Read the model definition and answer for the solid it produces. Units are mm, in the model's axes. A direction names the side the tool comes from. Give positions to 0.01 mm unless a question says otherwise; leave off trailing zeros. Write each loop counter-clockwise with the first axis right and the second up, starting at its lowest first coordinate (ties: lowest second). Pieces come first, ordered by that corner, then holes. Notation, with made-up numbers: M 26,-33 L 62,-33 A20 ccw 62,-17 Z; hole C 43.25,-17 d9. An arc over 180 degrees is marked long. Put each result on its own line as item: value.
from build123d import *

# Parameters (mm, degrees)
BOSS_EXTRUDE1_DEPTH = 10
SKETCH2_R           = 3
CUT_EXTRUDE1_DEPTH  = 34
SKETCH3_W           = 8.31174776
SKETCH3_H           = 3.43251071
BOSS_EXTRUDE2_DEPTH = 40
SKETCH4_R           = 2.5
CUT_EXTRUDE2_DEPTH  = 9.963348995


with BuildPart() as part:
    # Sketch1 → Boss-Extrude1 (new body)
    with BuildSketch(Plane.XY):
        with BuildLine():
            Line((0, 0), (38.333333333, 0))
            ThreePointArc((38.333333333, 0), (39.914472163, -0.25658351), (41.333333333, -1))
            Line((41.333333333, -1), (78.666666667, -29))
            ThreePointArc((78.666666667, -29), (80.085527837, -29.74341649), (81.666666667, -30))
            Line((81.666666667, -30), (100, -30))
            Line((100, -30), (100, -33))
            Line((100, -33), (81.666666667, -33))
            ThreePointArc((81.666666667, -33), (79.136844539, -32.589466384), (76.866666667, -31.4))
            Line((76.866666667, -31.4), (39.533333333, -3.4))
            ThreePointArc((39.533333333, -3.4), (38.965788865, -3.102633404), (38.333333333, -3))
            Line((38.333333333, -3), (0, -3))
            Line((0, -3), (0, 0))
        make_face()
    extrude(amount=BOSS_EXTRUDE1_DEPTH)

    # Sketch2 → Cut-Extrude1 (cut, through all)
    with BuildSketch(Plane(origin=(0, 0, 0), x_dir=(1, 0, 0), z_dir=(0, 1, 0))):
        with Locations((6.267592097, -5)):
            Circle(SKETCH2_R)
        with Locations((31.216017877, -5)):
            Circle(SKETCH2_R)
        with Locations((89.111430709, -5)):
            Circle(SKETCH2_R)
    extrude(amount=-CUT_EXTRUDE1_DEPTH, mode=Mode.SUBTRACT)

    # Sketch3 → Boss-Extrude2 (add)
    with BuildSketch(Plane.XZ.offset(33)):
        with Locations((95.527410175, 7.24709364)):
            Rectangle(SKETCH3_W, SKETCH3_H)
    extrude(amount=BOSS_EXTRUDE2_DEPTH)

    # Sketch4 → Cut-Extrude2 (cut, through all)
    with BuildSketch(Plane.XY.offset(8.963348995)):
        with Locations((95.527410175, -67.614542538)):
            Circle(SKETCH4_R)
    extrude(amount=-CUT_EXTRUDE2_DEPTH, mode=Mode.SUBTRACT)


solid = part.part
(1) Section A-A on z = 3.25 is taken. Determine the outline of the cut face in (x, y).
Result:
outline: M 0,-3 L 3.83,-3 L 3.83,0 L 0,0 Z; M 8.7,-3 L 28.78,-3 L 28.78,0 L 8.7,0 Z; M 33.65,-3 L 38.33,-3 A2 cw 39.53,-3.4 L 76.87,-31.4 A8 ccw 81.67,-33 L 86.67,-33 L 86.67,-30 L 81.67,-30 A5 cw 78.67,-29 L 41.33,-1 A5 ccw 38.33,0 L 33.65,0 Z; M 91.55,-33 L 100,-33 L 100,-30 L 91.55,-30 Z
(2) Section B-B on x = 89 is taken. Determine the outline of the cut face in (y, z).
Result:
outline: M -33,0 L -30,0 L -30,2 L -33,2 Z; M -33,8 L -30,8 L -30,10 L -33,10 Z
(3) Given pin 1 Ø0.6 at (x, z) = (92, 6) entering from +Y; pin 2 Ø9 at (x, y) = (96.5, -49) entering from -Z; pin 3 Ø3 at (y, z) = (-28, 6.5) entering from +X, each flat-ended and moving along its own axis, determine where each tip first touches the part or whether it passes through.
Result:
pin 1: stops at y = -30
pin 2: stops at z = 5.53
pin 3: stops at x = 79.49
(4) Straight lines are drawn through the part: line 1 along X through (y, z) = (-1.05, 5); line 2 along Y through (x, z) = (24, 5.75); line 3 along X through (y, z) = (-1.95, 5). For each, find the intervals that lie inside material, in ascending order. Write a range as from..to.
Result:
line 1: x = 0..3.27, 9.27..28.22, 34.22..41.4
line 2: y = -3..0
line 3: x = 0..3.27, 9.27..28.22, 34.22..42.6
(5) Which of the six approach directions +Z, -Z, +X, -X, +Y, -Y give full straight-line access (tool end or side, diameter ignored) to faces 1 (the face through (95, -53, 8.963)), 2 (the face through (99.683, -53, 7)), 3 (the face through (95, -53, 5.531)), 4 (the face through (93, -30, 5))?
Result:
face 1: +Z, +X, -X, -Y
face 2: +Z, -Z, +X, -Y
face 3: -Z, +X, -X, -Y
face 4: +Z, -Z, +X, +Y
(6) Section C-C on y = -15 is taken. Determine the outline of the cut face in (x, z), and give its area (3 significant figures).
Result:
outline: M 55,0 L 60,0 L 60,10 L 55,10 Z
area: 50.0 mm²
(7) Section D-D on x = 25.5 is taken. Determine the outline of the cut face in (y, z).
Result:
outline: M -3,0 L 0,0 L 0,10 L -3,10 Z
(8) For a pull along Y with two mould halves and no side action, classify faces 5 (the face through (58.461, -17.596, 4.93)), 6 (the face through (39.89, -0.25, 4.93)), 7 (the face through (96.681, -69.832, 7.271)) as +Y half, -Y half, draft (parallel to the pull), parting line (faces both ways), or undercut.
Result:
face 5: -Y half
face 6: +Y half
face 7: undercut
